from build123d import *

# Parameters (mm, degrees)
ESQUISSE1_R             = 76
BOSS_EXTRU_1_DEPTH      = 5
ESQUISSE2_R             = 2.1
ENL_V_MAT_EXTRU_1_DEPTH = 10
ESQUISSE4_R             = 1.5
ESQUISSE4_R_2           = 2
ENL_V_MAT_EXTRU_2_DEPTH = 10
ESQUISSE5_R             = 76
ESQUISSE5_R_2           = 68.5
BOSS_EXTRU_2_DEPTH      = 7
ESQUISSE6_R             = 4.5
ENL_V_MAT_EXTRU_3_DEPTH = 7
ESQUISSE7_R             = 71.5
ENL_V_MAT_EXTRU_4_DEPTH = 7
ESQUISSE8_W             = 3.5
ESQUISSE8_H             = 6.5
ENL_V_MAT_EXTRU_5_DEPTH = 4
ESQUISSE10_R            = 2.55
ENL_V_MAT_EXTRU_6_DEPTH = 4


with BuildPart() as part:
    # Esquisse1 → Boss.-Extru.1 (new body)
    with BuildSketch(Plane.XY):
        Circle(ESQUISSE1_R)
    extrude(amount=BOSS_EXTRU_1_DEPTH)

    # Esquisse2 → Enlèv. mat.-Extru.1 (cut)
    with BuildSketch(Plane.XY.offset(5)):
        with Locations((-55.497382355, 18.021183418)):
            Circle(ESQUISSE2_R)
        with Locations((-34.305739626, 47.199986533)):
            Circle(ESQUISSE2_R)
        with Locations((-0.010470369, 58.349999061)):
            Circle(ESQUISSE2_R)
        with Locations((34.288798212, 47.212295191)):
            Circle(ESQUISSE2_R)
        with Locations((55.49091131, 18.041099245)):
            Circle(ESQUISSE2_R)
        with Locations((55.497382355, -18.021183418)):
            Circle(ESQUISSE2_R)
        with Locations((34.305739626, -47.199986533)):
            Circle(ESQUISSE2_R)
        with Locations((0.010470369, -58.349999061)):
            Circle(ESQUISSE2_R)
        with Locations((-34.288798212, -47.212295191)):
            Circle(ESQUISSE2_R)
        with Locations((-55.49091131, -18.041099245)):
            Circle(ESQUISSE2_R)
        with Locations((-11.082204515, -21.759702771)):
            Circle(ESQUISSE2_R)
        with Locations((-21.759702771, 11.082204515)):
            Circle(ESQUISSE2_R)
        with Locations((11.082204515, 21.759702771)):
            Circle(ESQUISSE2_R)
        with Locations((21.759702771, -11.082204515)):
            Circle(ESQUISSE2_R)
    extrude(amount=-ENL_V_MAT_EXTRU_1_DEPTH, mode=Mode.SUBTRACT)

    # Esquisse4 → Enlèv. mat.-Extru.2 (cut)
    with BuildSketch(Plane.XY.offset(5)):
        with Locations((-20.704138623, -63.720786592)):
            Circle(ESQUISSE4_R)
        with Locations((-67, 0)):
            Circle(ESQUISSE4_R)
        with Locations((-20.704138623, 63.720786592)):
            Circle(ESQUISSE4_R)
        with Locations((54.204138623, 39.381611904)):
            Circle(ESQUISSE4_R)
        with Locations((54.204138623, -39.381611904)):
            Circle(ESQUISSE4_R)
        Circle(ESQUISSE4_R_2)
    extrude(amount=-ENL_V_MAT_EXTRU_2_DEPTH, mode=Mode.SUBTRACT)

    # Esquisse5 → Boss.-Extru.2 (add)
    with BuildSketch(Plane.XY.offset(5)):
        Circle(ESQUISSE5_R)
        with Locations(Location((0, 0, 0), (0, 0, 179.999985351))):
            Circle(ESQUISSE5_R_2, mode=Mode.SUBTRACT)
    extrude(amount=BOSS_EXTRU_2_DEPTH)

    # Esquisse6 → Enlèv. mat.-Extru.3 (cut)
    with BuildSketch(Plane.XY.offset(12)):
        with Locations((-20.704138623, 63.720786592)):
            Circle(ESQUISSE6_R)
        with Locations((54.204138623, 39.381611904)):
            Circle(ESQUISSE6_R)
        with Locations((54.204138623, -39.381611904)):
            Circle(ESQUISSE6_R)
        with Locations((-20.704138623, -63.720786592)):
            Circle(ESQUISSE6_R)
        with Locations((-67, 0)):
            Circle(ESQUISSE6_R)
    extrude(amount=-ENL_V_MAT_EXTRU_3_DEPTH, mode=Mode.SUBTRACT)

    # Esquisse7 → Enlèv. mat.-Extru.4 (cut)
    with BuildSketch(Plane.XY.offset(12)):
        Circle(ESQUISSE7_R)
    extrude(amount=-ENL_V_MAT_EXTRU_4_DEPTH, mode=Mode.SUBTRACT)

    # Esquisse8 → Enlèv. mat.-Extru.5 (cut)
    with BuildSketch(Plane.XY.offset(5)):
        with Locations((-18.309702771, -6.25)):
            Rectangle(ESQUISSE8_W, ESQUISSE8_H)
    extrude(amount=-ENL_V_MAT_EXTRU_5_DEPTH, mode=Mode.SUBTRACT)

    # Esquisse10 → Enlèv. mat.-Extru.6 (cut)
    with BuildSketch(Plane(origin=(0, 0, 0), x_dir=(-1, 0, 0), z_dir=(0, 0, -1))):
        with Locations((-67, 0)):
            Circle(ESQUISSE10_R)
    extrude(amount=-ENL_V_MAT_EXTRU_6_DEPTH, mode=Mode.SUBTRACT)


solid = part.part
Design review of the part built by this model. Coordinates are the model's own, in mm. A direction names the side the tool comes from. Round coordinates to 2 decimals unless told otherwise and drop trailing zeros. Loops run counter-clockwise (first coordinate to the right, second up) from the corner with the lowest first, then second, coordinate; pieces in that order, holes last. Notation, with made-up numbers: (70, 61) - (114, 61) arc R21 ccw to (114, 79) - close; hole circle Ø4 at (68.25, 88.25). An arc over 180 degrees is marked (long way). One line per item, written item: value. Start each with the question number.
1) Consider section C-C on z = 8. Give the boundary of the cut face in (x, y), then the cut area to 3 significant figures.
2) Insertion check: pin 1 Ø6 at (y, z) = (57, 10) entering from +X; pin 2 Ø2.5 at (x, y) = (-67, 0) entering from -Z; pin 3 Ø3 at (x, z) = (-51, 6.5) entering from +Y; pin 4 Ø3 at (y, z) = (-7, 3.5) entering from +X. Each pin has a flat end and moves straight along its axis. Give the tip position at first contact, or say it passes through.
3) Consider section B-B on x = 0. Give the boundary of the cut face in (y, z), then the cut area to 3 significant figures.
4) To check wall thickness, follow L1, parallel to X at y = 46.5, z = 3.75; L2, parallel to X at y = 48.5, z = 1.75; L3, parallel to Z at x = 34, y = 15.5. State the ranges of each line that lie inside material, in increasing order. Write a range as from..to.
5) Consider section D-D on x = 67. Give the boundary of the cut face in (y, z), then the cut area to 3 significant figures.
6) Consider section A-A on y = -58.35. Give the boundary of the cut face in (x, z).
7) Draft analysis for pull direction X (two halves, no side actions). For faces 1 (the flat face through (56, -45, 12)), 2 (the cylindrical face through (35.069, -67.425, 5.916)), 3 (the cylindrical face through (9.534, 23.179, 2.535)), 4 (the cylindrical face through (-52.7, 48.32, 8.55)), state which applies: +X half, -X half, draft (parallel to the pull), parting line (faces both ways), or undercut.
8) For faces 5 (the flat face through (67, 0, 4)), 6 (the flat face through (-18, -9.5, 3)), 7 (the cylindrical face through (23.763, -10.451, 2.535)), list the 3-axis set-ups (+Z, -Z, +X, -X, +Y, -Y) from which the entire face can be reached by the end or side of a thin tool; tool diameter is ignored.
Reported:
1. outline: circle Ø152 at (0, 0); hole circle Ø143 at (0, 0)
1. area: 2,090 mm^2
2. pin 1: stops at x = 53.48
2. pin 2: passes through
2. pin 3: stops at y = 57.67
2. pin 4: stops at x = 75.8
3. outline: (-76, 0) - (-60.45, 0) - (-60.45, 5) - (-71.5, 5) - (-71.5, 12) - (-76, 12) - close; (-56.25, 0) - (-2, 0) - (-2, 5) - (-56.25, 5) - close; (2, 0) - (56.25, 0) - (56.25, 5) - (2, 5) - close; (60.45, 0) - (76, 0) - (76, 12) - (71.5, 12) - (71.5, 5) - (60.45, 5) - close
3. area: 761 mm^2
4. L1: x = -60.11..-36.29, -32.33..32.31, 36.26..60.11
4. L2: x = -58.51..-35.95, -32.66..32.63, 35.95..58.51
4. L3: z = 0..5
5. outline: (-35.87, 0) - (-2.55, 0) - (-2.55, 4) - (2.55, 4) - (2.55, 0) - (35.87, 0) - (35.87, 12) - (24.96, 12) - (24.96, 5) - (-24.96, 5) - (-24.96, 12) - (-35.87, 12) - close
5. area: 491 mm^2
6. outline: (-48.7, 0) - (-2.09, 0) - (-2.09, 5) - (-41.32, 5) - (-41.32, 12) - (-48.7, 12) - close; (2.11, 0) - (48.7, 0) - (48.7, 12) - (41.32, 12) - (41.32, 5) - (2.11, 5) - close
7. face 1: draft
7. face 2: parting line
7. face 3: undercut
7. face 4: undercut
8. face 5: -Z
8. face 6: +Z
8. face 7: +Z, -Z
